Verification items for the finished model (mm, model axes). A direction names the side the tool comes from. Coordinates: 2 decimals unless noted, no trailing zeros. Write each loop counter-clockwise with the first axis right and the second up, starting at its lowest first coordinate (ties: lowest second). Pieces come first, ordered by that corner, then holes. Notation, with made-up numbers: (41.5, 22.5) -> (96.5, 22.5) arc R27 ccw to (96.5, 46.5) -> close; hole circle Ø4 at (46, -30). An arc over 180 degrees is marked (long way). Write each question's results on one line, items separated by ' | '. Start each with the question number.
from build123d import *

# Parameters (mm, degrees)
F0_R      = 17.5
F1_DEPTH  = 30
F2_SIZE   = 5
F3_R      = 8.75
F1_FACE_R = 12.5
F4_DEPTH  = 55
F5_SIZE   = 12.5


with BuildPart() as f1:
    # F0 (on Front) → F1 (new body)
    with BuildSketch(Plane.XZ):
        Circle(F0_R)
    extrude(amount=F1_DEPTH)

    # F2
    f2_edges = [f1.edges().sort_by_distance(p)[0] for p in [
        (17.5, -15, 0),
        (-17.5, 0, 0),
        (-17.5, -30, 0),
    ]]
    chamfer(f2_edges, length=F2_SIZE)

    # F3 (on Front) + F1_face (on face) → F4 (join)
    with BuildSketch(Plane.XZ):
        Circle(F3_R)
    with BuildSketch(Plane.XZ.offset(30)):
        Circle(F1_FACE_R)
    extrude(amount=F4_DEPTH)

    # F5
    f5_edges = [f1.edges().sort_by_distance(p)[0] for p in [
        (-12.5, -85, 0),
    ]]
    chamfer(f5_edges, length=F5_SIZE)


solid = f1.part
1. Tool access check on faces 1 (the cylindrical face through (11.923, -50.952, 3.755)), 2 (the flat face through (0, 0, 0)). Record the directions out of +Z, -Z, +X, -X, +Y, -Y that give a thin tool (end or side, any length) a straight path to the whole face; none if there is none.
2. Sectioned sample at B-B on y = -75. Record the cut outline in (x, z).
3. Depth check by flat-ended pin: pin 1 Ø3 at (x, z) = (-3, -1.5) entering from -Y; pin 2 Ø10 at (x, y) = (12.5, -21.5) entering from -Z; pin 3 Ø2 at (x, y) = (11, -29) entering from -Z (3 decimals); pin 4 Ø6 at (x, z) = (-10, -10.5) entering from +Y. Enter the tip coordinate at first touch or a pass-through.
4. Sectioned sample at A-A on y = -15. Record the cut outline in (x, z), plus the area to 3 significant figures.
5. Material ranges on probe 1 along Y at (x, z) = (8, 11); probe 2 along Y at (x, z) = (1, 16); probe 3 along Z at (x, y) = (-13, -6), recorded low to high. Write a range as from..to.
Computed values:
1) face 1: -Y | face 2: +Z, -Z, +X, -X, +Y
2) outline: circle Ø20 at (0, 0)
3) pin 1: stops at y = -83.15 | pin 2: stops at z = -15.81 | pin 3: stops at z = -9.815 | pin 4: stops at y = 0
4) outline: circle Ø35 at (0, 0) | area: 962 mm^2
5) probe 1: y = -28.9..-1.1 | probe 2: y = -26.47..-3.53 | probe 3: z = -11.72..11.72
